```python
from build123d import *

# Parameters (mm, degrees)
SKETCH_1_W             = 61.5
SKETCH_1_H             = 20
EXTRUDE_1_DEPTH        = 3
EXTRUDE_2_DEPTH        = 3
PATTERN_LINEAR_1_COUNT = 16
PATTERN_LINEAR_1_PITCH = 3.141592654
CUT_EXTRUDE_1_REACH    = 35.236
SKETCH_3_R             = 1.65
CUT_EXTRUDE_2_REACH    = 35.236
SKETCH_4_R             = 1.65


with BuildPart() as part:
    # 草圖1 → 填料-伸長1 (new body)
    with BuildSketch(Plane.XY):
        Rectangle(SKETCH_1_W, SKETCH_1_H)
    extrude(amount=EXTRUDE_1_DEPTH)

    # 草圖2 → 填料-伸長2 (add)
    with BuildSketch(Plane.XY.offset(3)):
        Polygon((-29.75, 10), (-28.931066973, 12.25), (-28.088211111, 12.25), (-27.269278084, 10), align=None)
    extrude_2 = extrude(amount=-EXTRUDE_2_DEPTH)

    # 直線複製排列1: 填料-伸長2 ×16
    with Locations(*[(i * PATTERN_LINEAR_1_PITCH, 0, 0) for i in range(1, PATTERN_LINEAR_1_COUNT)]):
        add(extrude_2)

    # 草圖3 → 除料-伸長1 (cut, up to next)
    with BuildSketch(Plane.XY.offset(3), mode=Mode.PRIVATE) as cut_extrude_1_sk1:
        with Locations((-21.75, 6)):
            Circle(SKETCH_3_R)
    cut_extrude_1_tool1 = extrude(cut_extrude_1_sk1.sketch, amount=-CUT_EXTRUDE_1_REACH, mode=Mode.PRIVATE) & part.part
    # 草圖3 → 除料-伸長1 (cut, up to next)
    with BuildSketch(Plane.XY.offset(3), mode=Mode.PRIVATE) as cut_extrude_1_sk2:
        with Locations((-13.75, 6)):
            Circle(SKETCH_3_R)
    cut_extrude_1_tool2 = extrude(cut_extrude_1_sk2.sketch, amount=-CUT_EXTRUDE_1_REACH, mode=Mode.PRIVATE) & part.part
    # 草圖3 → 除料-伸長1 (cut, up to next)
    with BuildSketch(Plane.XY.offset(3), mode=Mode.PRIVATE) as cut_extrude_1_sk3:
        with Locations((-21.75, -6)):
            Circle(SKETCH_3_R)
    cut_extrude_1_tool3 = extrude(cut_extrude_1_sk3.sketch, amount=-CUT_EXTRUDE_1_REACH, mode=Mode.PRIVATE) & part.part
    # 草圖3 → 除料-伸長1 (cut, up to next)
    with BuildSketch(Plane.XY.offset(3), mode=Mode.PRIVATE) as cut_extrude_1_sk4:
        with Locations((-13.75, -6)):
            Circle(SKETCH_3_R)
    cut_extrude_1_tool4 = extrude(cut_extrude_1_sk4.sketch, amount=-CUT_EXTRUDE_1_REACH, mode=Mode.PRIVATE) & part.part
    add(cut_extrude_1_tool1.solids().sort_by_distance((-21.75, 6, 3))[0], mode=Mode.SUBTRACT)
    add(cut_extrude_1_tool2.solids().sort_by_distance((-13.75, 6, 3))[0], mode=Mode.SUBTRACT)
    add(cut_extrude_1_tool3.solids().sort_by_distance((-21.75, -6, 3))[0], mode=Mode.SUBTRACT)
    add(cut_extrude_1_tool4.solids().sort_by_distance((-13.75, -6, 3))[0], mode=Mode.SUBTRACT)

    # 草圖4 → 除料-伸長2 (cut, up to next)
    with BuildSketch(Plane.XY.offset(3), mode=Mode.PRIVATE) as cut_extrude_2_sk1:
        with Locations((25.75, 5)):
            Circle(SKETCH_4_R)
    cut_extrude_2_tool1 = extrude(cut_extrude_2_sk1.sketch, amount=-CUT_EXTRUDE_2_REACH, mode=Mode.PRIVATE) & part.part
    # 草圖4 → 除料-伸長2 (cut, up to next)
    with BuildSketch(Plane.XY.offset(3), mode=Mode.PRIVATE) as cut_extrude_2_sk2:
        with Locations((10.75, 5)):
            Circle(SKETCH_4_R)
    cut_extrude_2_tool2 = extrude(cut_extrude_2_sk2.sketch, amount=-CUT_EXTRUDE_2_REACH, mode=Mode.PRIVATE) & part.part
    # 草圖4 → 除料-伸長2 (cut, up to next)
    with BuildSketch(Plane.XY.offset(3), mode=Mode.PRIVATE) as cut_extrude_2_sk3:
        with Locations((25.75, -5)):
            Circle(SKETCH_4_R)
    cut_extrude_2_tool3 = extrude(cut_extrude_2_sk3.sketch, amount=-CUT_EXTRUDE_2_REACH, mode=Mode.PRIVATE) & part.part
    # 草圖4 → 除料-伸長2 (cut, up to next)
    with BuildSketch(Plane.XY.offset(3), mode=Mode.PRIVATE) as cut_extrude_2_sk4:
        with Locations((10.75, -5)):
            Circle(SKETCH_4_R)
    cut_extrude_2_tool4 = extrude(cut_extrude_2_sk4.sketch, amount=-CUT_EXTRUDE_2_REACH, mode=Mode.PRIVATE) & part.part
    add(cut_extrude_2_tool1.solids().sort_by_distance((25.75, 5, 3))[0], mode=Mode.SUBTRACT)
    add(cut_extrude_2_tool2.solids().sort_by_distance((10.75, 5, 3))[0], mode=Mode.SUBTRACT)
    add(cut_extrude_2_tool3.solids().sort_by_distance((25.75, -5, 3))[0], mode=Mode.SUBTRACT)
    add(cut_extrude_2_tool4.solids().sort_by_distance((10.75, -5, 3))[0], mode=Mode.SUBTRACT)


solid = part.part
```
Geometry: final body of the model. Coordinates: model frame, mm. A direction names the side the tool comes from. Round coordinates to 2 decimals unless told otherwise and drop trailing zeros. Loops run counter-clockwise (first coordinate to the right, second up) from the corner with the lowest first, then second, coordinate; pieces in that order, holes last.
Item 1: Reachability of faces 3 (the flat face through (-2.55, 11.14, 1.52)), 4 (the cylindrical face through (12.274, -5.632, 1.521)) from +Z, -Z, +X, -X, +Y, -Y: full face, straight path, thin tool, end or side. Return the list, or none.
Checked values:
face 3: +Z, -Z, +Y
face 4: +Z, -Z
Item 2: Line query: L1, parallel to Y at x = 25.75, z = 2; L2, parallel to X at y = 3.75, z = 0.2; L3, parallel to X at y = 3.5, z = 2. Output: solid intervals per line, ascending.
Checked values:
L1: y = -10 to -6.65, -3.35 to 3.35, 6.65 to 10
L2: x = -30.75 to 9.67, 11.83 to 24.67, 26.83 to 30.75
L3: x = -30.75 to 10.06, 11.44 to 25.06, 26.44 to 30.75
Item 3: Section A-A, the plane y = 5. Output: boundary loops of the cut face in (x, z).
Checked values:
outline: (-30.75, 0) - (-23.06, 0) - (-23.06, 3) - (-30.75, 3) - close; (-20.44, 0) - (-15.06, 0) - (-15.06, 3) - (-20.44, 3) - close; (-12.44, 0) - (9.1, 0) - (9.1, 3) - (-12.44, 3) - close; (12.4, 0) - (24.1, 0) - (24.1, 3) - (12.4, 3) - close; (27.4, 0) - (30.75, 0) - (30.75, 3) - (27.4, 3) - close
Item 4: Contact query for flat-ended pins moving along their axis: P1, Ø0.5, axis at x = 4.5, z = 1.5, coming from the +Y side; P2, Ø3, axis at x = 25.75, y = 5, coming from the -Z side (3 decimals). Output: stop coordinate, or through.
Checked values:
P1: stops at y = 10
P2: passes through
Item 5: Section B-B, the plane z = 1.85. State how many separate pieces and enclosed holes the cut face has, plus the area to 3 significant figures.
Checked values:
separate pieces: 1
enclosed holes: 8
area: 1,220 mm2
Item 6: Mould query, pull axis X, two halves, no side actions, for faces 1 (the flat face through (-8.835, 11.141, 1.521)), 2 (the flat face through (25, 10, 1)). Classes: released by +X, released by -X, zero draft, split by the parting line, or undercut.
Checked values:
face 1: undercut
face 2: zero draft
